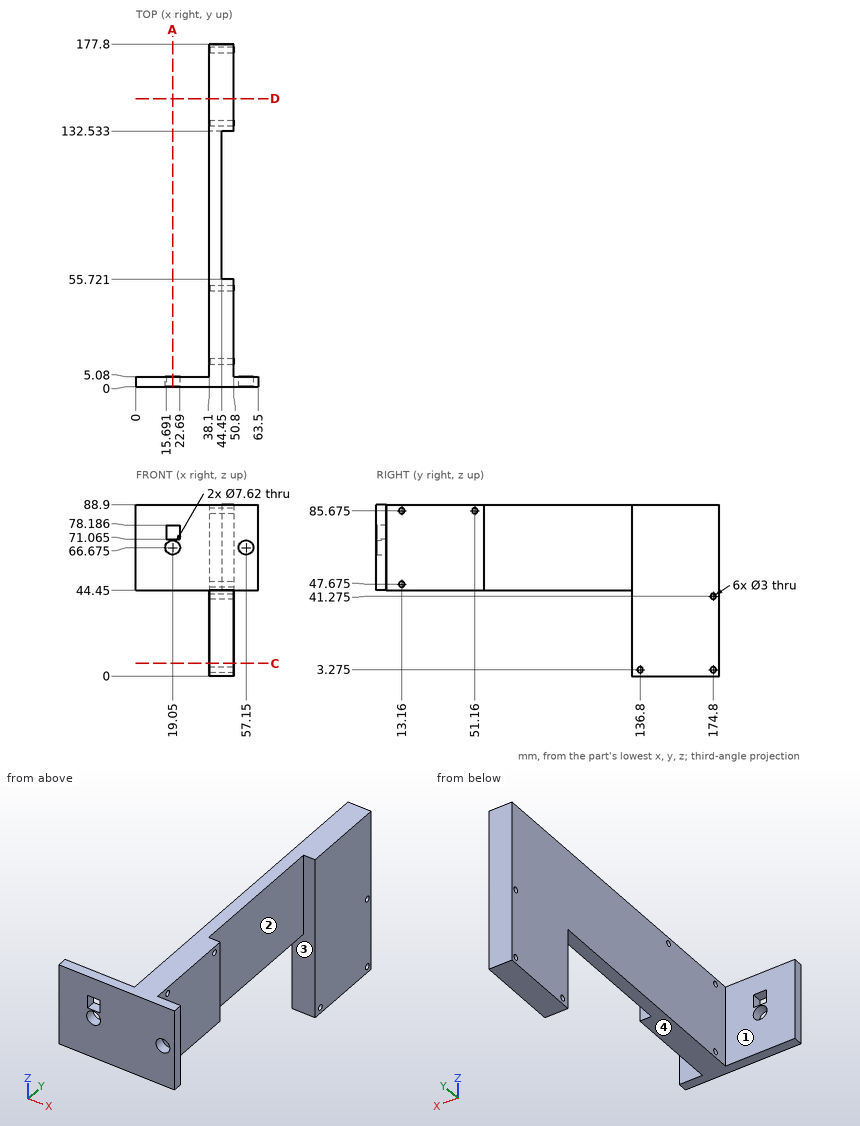
The drawing under review shows one solid part. Ordinate dimensions are in mm from its lowest x, y, z. A direction names the side the tool comes from. Coordinates: 2 decimals unless noted, no trailing zeros. Write each loop counter-clockwise with the first axis right and the second up, starting at its lowest first coordinate (ties: lowest second). Pieces come first, ordered by that corner, then holes.
1) Insertion check: pin 1 (14 mm diameter, centred on x = 58, z = 71, fed in from +Y); pin 2 (4 mm diameter, centred on y = 136.8, z = 3.275, fed in from -X); pin 3 (2.5 mm diameter, centred on y = 13.16, z = 47.68, fed in from -X); pin 4 (19 mm diameter, centred on x = 35, y = 82, fed in from -Z). Each pin has a flat end and moves straight along its axis. Give the tip position at first contact, or say it passes through.
2) Add section D-D (y = 149.5). Write out the cut boundary in (x, z).
3) Machinability: for the marked faces 1, 2, 3 and 4, which of the approach directions +Z, -Z, +X, -X, +Y, -Y give a long, thin tool a straight path to every point of the face, cutting with its end or side? Answer none if there is none.
4) Add section A-A (x = 19.05). State how many separate pieces and enclosed holes the cut face has, plus the area to 3 significant figures.
5) Add section C-C (z = 6.5). Write out the cut boundary in (x, y), plus the area to 3 significant figures.
6) To check wall thickness, follow L1, parallel to Z at x = 40.5, y = 14; L2, parallel to Z at x = 43, y = 174 (1 decimal); L3, parallel to Y at x = 45.5, z = 46.5 (1 decimal). State the ranges of each line that lie inside material, in increasing order.
Check result:
1. pin 1: stops at y = 5.08
1. pin 2: stops at x = 38.1
1. pin 3: passes through
1. pin 4: stops at z = 44.45
2. outline: (38.1, 0) - (50.8, 0) - (50.8, 88.9) - (38.1, 88.9) - close
3. face 1: +Z, -Z, -X, +Y
3. face 2: +Z, -Z, +X
3. face 3: -Z, +X
3. face 4: -Z, +X, -X, -Y
4. separate pieces: 3
4. enclosed holes: 0
4. area: 151 mm2
5. outline: (38.1, 132.53) - (50.8, 132.53) - (50.8, 177.8) - (38.1, 177.8) - close
5. area: 575 mm2
6. L1: z = 44.45 to 46.43, 48.92 to 84.43, 86.92 to 88.9
6. L2: z = 0 to 2, 4.5 to 40, 42.5 to 88.9
6. L3: y = 0 to 12.2, 14.1 to 55.7, 132.5 to 177.8
